Geometry check sheet. Reference: the model listing, model coordinates, mm. Coordinates: 2 decimals unless noted, no trailing zeros. Loops run counter-clockwise (first coordinate to the right, second up) from the corner with the lowest first, then second, coordinate; pieces in that order, holes last. Notation, with made-up numbers: (89.25, 71) -> (129.25, 71) arc R23 ccw to (129.25, 106) -> close; hole circle Ø9 at (61, 41). An arc over 180 degrees is marked (long way). Answer as a JSON object with one key per item and string values.
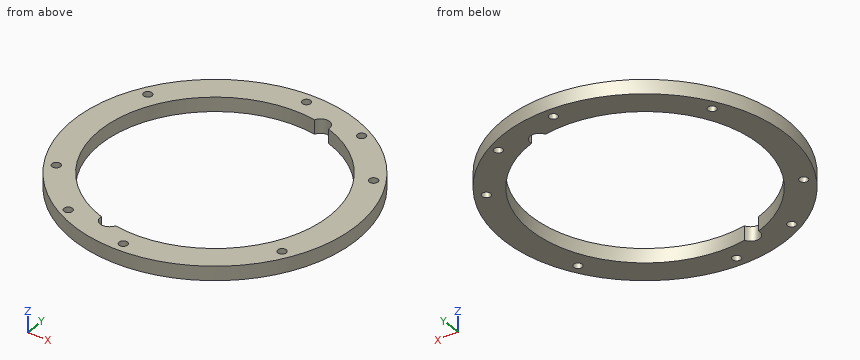
from build123d import *

# Parameters (mm, degrees)
ESQUISSE1_R        = 50
ESQUISSE1_R_2      = 1.5
BOSS_EXTRU_1_DEPTH = 5
SKETCH4_R          = 1.5
CUT_EXTRUDE4_DEPTH = 10
SKETCH5_R          = 40.5
CUT_EXTRUDE5_DEPTH = 10
SKETCH6_R          = 3.2
CUT_EXTRUDE6_DEPTH = 10


with BuildPart() as part:
    # Esquisse1 → Boss.-Extru.1 (new body)
    with BuildSketch(Plane.XY):
        Circle(ESQUISSE1_R)
        with Locations((-40.096976195, -23.15)):
            Circle(ESQUISSE1_R_2, mode=Mode.SUBTRACT)
        with Locations((-40.096976195, 23.15)):
            Circle(ESQUISSE1_R_2, mode=Mode.SUBTRACT)
        with Locations((0, 46.3)):
            Circle(ESQUISSE1_R_2, mode=Mode.SUBTRACT)
        with Locations((40.096976195, 23.15)):
            Circle(ESQUISSE1_R_2, mode=Mode.SUBTRACT)
        with Locations((40.096976195, -23.15)):
            Circle(ESQUISSE1_R_2, mode=Mode.SUBTRACT)
        with Locations((0, -46.3)):
            Circle(ESQUISSE1_R_2, mode=Mode.SUBTRACT)
    extrude(amount=BOSS_EXTRU_1_DEPTH)

    # Sketch4 → Cut-Extrude4 (cut)
    with BuildSketch(Plane.XY.offset(5)):
        with Locations((-23.5, -40.703193978)):
            Circle(SKETCH4_R)
        with Locations((23.5, 40.703193978)):
            Circle(SKETCH4_R)
    extrude(amount=-CUT_EXTRUDE4_DEPTH, mode=Mode.SUBTRACT)

    # Sketch5 → Cut-Extrude5 (cut)
    with BuildSketch(Plane.XY.offset(5)):
        Circle(SKETCH5_R)
    extrude(amount=-CUT_EXTRUDE5_DEPTH, mode=Mode.SUBTRACT)

    # Sketch6 → Cut-Extrude6 (cut)
    with BuildSketch(Plane.XY.offset(5)):
        with Locations((10.352761804, 38.637033052)):
            Circle(SKETCH6_R)
        with Locations((-10.352761804, -38.637033052)):
            Circle(SKETCH6_R)
    extrude(amount=-CUT_EXTRUDE6_DEPTH, mode=Mode.SUBTRACT)


solid = part.part
1. Section check A-A, the plane x = 0. Record the boundary of the cut face in (y, z), then the cut area to 3 significant figures.
Evaluation:
{"outline": "(-50, 0) -> (-47.8, 0) -> (-47.8, 5) -> (-50, 5) -> close; (-44.8, 0) -> (-40.5, 0) -> (-40.5, 5) -> (-44.8, 5) -> close; (40.5, 0) -> (44.8, 0) -> (44.8, 5) -> (40.5, 5) -> close; (47.8, 0) -> (50, 0) -> (50, 5) -> (47.8, 5) -> close", "area": "65.0 mm^2"}
2. Section check D-D, the plane z = 0.95. State how many separate pieces and enclosed holes the cut face has, then the cut area to 3 significant figures.
Evaluation:
{"separate pieces": "1", "enclosed holes": "9", "area": "2,620 mm^2"}
3. Section check C-C, the plane x = 23.5. Record the boundary of the cut face in (y, z).
Evaluation:
{"outline": "(-44.13, 0) -> (-32.98, 0) -> (-32.98, 5) -> (-44.13, 5) -> close; (32.98, 0) -> (39.2, 0) -> (39.2, 5) -> (32.98, 5) -> close; (42.2, 0) -> (44.13, 0) -> (44.13, 5) -> (42.2, 5) -> close"}
4. Depth check by flat-ended pin: P1, Ø3, axis at y = -32.5, z = 4, coming from the +X side; P2, Ø1.8, axis at x = -40.1, y = -23.15, coming from the -Z side; P3, Ø2, axis at y = -9, z = 4, coming from the -X side; P4, Ø1.5, axis at x = 0.5, z = 4, coming from the +Y side. Enter the tip coordinate at first touch or a pass-through.
Evaluation:
{"P1": "stops at x = 39.23", "P2": "passes through", "P3": "stops at x = -49.36", "P4": "stops at y = 50"}
5. Section check B-B, the plane y = 0. Record the boundary of the cut face in (x, z).
Evaluation:
{"outline": "(-50, 0) -> (-40.5, 0) -> (-40.5, 5) -> (-50, 5) -> close; (40.5, 0) -> (50, 0) -> (50, 5) -> (40.5, 5) -> close"}
6. Thickness scan on probe 1 along Y at (x, z) = (0, 2.95); probe 2 along X at (y, z) = (-23, 3.8); probe 3 along X at (y, z) = (0.5, 2.45). Record the ranges inside material, lowest first. Write a range as from..to.
Evaluation:
{"probe 1": "y = -50..-47.8, -44.8..-40.5, 40.5..44.8, 47.8..50", "probe 2": "x = -44.4..-41.59, -38.6..-33.34, 33.34..38.6, 41.59..44.4", "probe 3": "x = -50..-40.5, 40.5..50"}
